Could you check a few things on this model? Use its own coordinates, in mm. Face numbers are marked on the shaded views. A direction names the side the tool comes from. Round coordinates to 2 decimals unless told otherwise and drop trailing zeros. Write each loop counter-clockwise with the first axis right and the second up, starting at its lowest first coordinate (ties: lowest second). Pieces come first, ordered by that corner, then holes. Notation, with made-up numbers: (8.25, 50.25) - (21.25, 50.25) arc R27 ccw to (21.25, 88.25) - close; hole circle Ø7 at (38, 28.25). An arc over 180 degrees is marked (long way). Put each result on its own line as item: value.
Autodesk Fusion 360 part; units mm, degrees
sketch "Sketch1" plane through (0, 0, 0) normal (0, 1, 0) x (1, 0, 0)
  line L0 (0, 0) -> (5.5, 0)
  line L1 (0, -3.5) -> (2.625, -3.5)
  line L2 (2.625, -3.5) -> (5.5, 0)
  line L3 (0, -1.75) -> (0, -22.5)
  line L4 (0, -3.5) -> (-2.625, -3.5)
  line L5 (-2.625, -3.5) -> (-5.5, 0)
  line L6 (0, 0) -> (-5.5, 0)
  line L7 (-4.5, -1.2174) -> (-4.5, 0)
  line L8 (4.5, -1.2174) -> (4.5, 0)
  dimension "d1" = 5.5
  dimension "d2" = 2.625
  dimension "d3" = 3.5
  dimension "d16" = 4.5
extrude "Extrude1" add sketch "Sketch1" along normal blind 38 contours L0 L1 L2 L4 L5 L6 L7 L8
sketch "Sketch2" plane through (0, 0, 3.5) normal (0, 0, 1) x (-1, 0, 0)
  line L0 (2.625, 0) -> (-2.625, 0)
  line L1 (-2.625, 0) -> (-2.625, -38)
  line L2 (-2.625, -38) -> (2.625, -38)
  line L3 (2.625, -38) -> (2.625, 0)
  line L4 (0, -38) -> (0, 0) construction
  line L5 (2.74, -29.9181) -> (0, -28.3361)
  line L6 (0, -28.3361) -> (-2.74, -29.9181)
  line L7 (-2.74, -29.9181) -> (-2.74, -33.0819)
  line L8 (-2.74, -33.0819) -> (0, -34.6639)
  line L9 (0, -34.6639) -> (2.74, -33.0819)
  line L10 (2.74, -33.0819) -> (2.74, -29.9181)
  line L11 (2.74, -4.9181) -> (0, -3.3361)
  line L12 (0, -3.3361) -> (-2.74, -4.9181)
  line L13 (-2.74, -4.9181) -> (-2.74, -8.0819)
  line L14 (-2.74, -8.0819) -> (0, -9.6639)
  line L15 (0, -9.6639) -> (2.74, -8.0819)
  line L16 (2.74, -8.0819) -> (2.74, -4.9181)
  point P0 (0, -31.5)
  point P1 (0, -6.5)
  dimension "d6" = 2.74
  dimension "d7" = 2.74
  dimension "d8" = 25
  dimension "d9" = 6.5
extrude "Extrude2" cut sketch "Sketch2" against normal blind 2.5 contours L1 L3 L11 L12 L14 L15 | L1 L3 L5 L6 L8 L9
hole "Hole1" at (0, 31.5, 3.5) at (0, 6.5, 3.5) direction (0, 0, -1) diameter 3.4 depth 16 tip angle 118
equation "d2 = ( 5.25 / 2 ) * 1 mm"
equation "d6 = ( 5.48 / 2 ) * 1 mm"
equation "d7 = ( 5.48 / 2 ) * 1 mm"
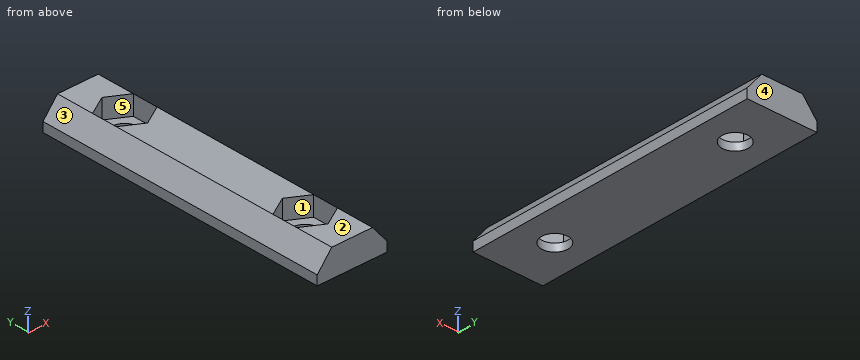
(1) Please list where these lines run through material, in increasing order: probe 1 along Y at (x, z) = (0, 0.5); probe 2 along Y at (x, z) = (0.75, 0.6); probe 3 along X at (y, z) = (31.5, 0.5). Write a range as from..to.
Values found:
probe 1: y = 0..4.8, 8.2..29.8, 33.2..38
probe 2: y = 0..4.97, 8.03..29.97, 33.03..38
probe 3: x = -4.5..-1.7, 1.7..4.5
(2) For the marked faces 1 and 2, which set-ups out of +Z, -Z, +X, -X, +Y, -Y let a thin tool reach every point of the face, with its end or its side?
Values found:
face 1: +Z
face 2: +Z, +X, -X, +Y, -Y
(3) If we mould it in two halves opening along X, with no side actions, what happens to the marked faces 3, 4 and 5? For each: pulls with the +X half, pulls with the -X half, needs draft (parallel to the pull), parting line crosses it, or undercut.
Values found:
face 3: pulls with the -X half
face 4: needs draft
face 5: undercut
(4) Imagine slicing it at C-C, the plane z = 2.8. List the corners of the cut face in (x, y) for me (3 decimals), then the cut area to 3 significant figures.
Values found:
outline: (-3.2, 0) - (3.2, 0) - (3.2, 38) - (-3.2, 38) - close; hole (-2.625, 4.852) - (0, 3.336) - (2.625, 4.852) - (2.625, 8.148) - (0, 9.664) - (-2.625, 8.148) - close; hole (-2.625, 29.852) - (0, 28.336) - (2.625, 29.852) - (2.625, 33.148) - (0, 34.664) - (-2.625, 33.148) - close
area: 193 mm^2
(5) Imagine slicing it at A-A, the plane y = 6.5. List the corners of the cut face in (x, z) for me (3 decimals).
Values found:
outline: (-4.5, 0) - (-1.7, 0) - (-1.7, 1) - (-2.625, 1) - (-2.625, 3.5) - (-4.5, 1.217) - close; (1.7, 0) - (4.5, 0) - (4.5, 1.217) - (2.625, 3.5) - (2.625, 1) - (1.7, 1) - close
(6) I'm going to push flat-ended pins straight in: pin 1 (2 mm diameter, centred on y = 32, z = 2.5, fed in from -X); pin 2 (2 mm diameter, centred on x = 0, y = 31.5, fed in from +Z); pin 3 (1.2 mm diameter, centred on y = 31, z = 2.5, fed in from +X); pin 4 (2.5 mm diameter, centred on x = -1, y = 5.5, fed in from +Z). Where does each tip first touch, or does it pass through?
Values found:
pin 1: stops at x = -4.27
pin 2: passes through
pin 3: stops at x = 3.94
pin 4: stops at z = 1
(7) Imagine slicing it at D-D, the plane y = 25.5. List the corners of the cut face in (x, z) for me (3 decimals), then the cut area to 3 significant figures.
Values found:
outline: (-4.5, 0) - (4.5, 0) - (4.5, 1.217) - (2.625, 3.5) - (-2.625, 3.5) - (-4.5, 1.217) - close
area: 27.2 mm^2
(8) Imagine slicing it at B-B, the plane x = -0.75. List the corners of the cut face in (y, z) for me.
Values found:
outline: (0, 0) - (4.97, 0) - (4.97, 1) - (3.77, 1) - (3.77, 3.5) - (0, 3.5) - close; (8.03, 0) - (29.97, 0) - (29.97, 1) - (28.77, 1) - (28.77, 3.5) - (9.23, 3.5) - (9.23, 1) - (8.03, 1) - close; (33.03, 0) - (38, 0) - (38, 3.5) - (34.23, 3.5) - (34.23, 1) - (33.03, 1) - close
